from build123d import *

# Parameters (mm, degrees)
ESQUISSE2_W             = 100
ESQUISSE2_H             = 100
BOSS_EXTRU_1_DEPTH      = 100
ESQUISSE3_R             = 10
ENL_V_MAT_EXTRU_1_DEPTH = 101
ESQUISSE4_R             = 10
ENL_V_MAT_EXTRU_2_DEPTH = 101


with BuildPart() as part:
    # Esquisse2 → Boss.-Extru.1 (new body)
    with BuildSketch(Plane.XY):
        with Locations((-50, 50)):
            Rectangle(ESQUISSE2_W, ESQUISSE2_H)
    extrude(amount=BOSS_EXTRU_1_DEPTH)

    # Esquisse3 → Enlèv. mat.-Extru.1 (cut, through all)
    with BuildSketch(Plane.XY.offset(100)):
        with Locations((-50, 50)):
            Circle(ESQUISSE3_R)
    extrude(amount=-ENL_V_MAT_EXTRU_1_DEPTH, mode=Mode.SUBTRACT)

    # Esquisse4 → Enlèv. mat.-Extru.2 (cut, through all)
    with BuildSketch(Plane(origin=(0, 100, 0), x_dir=(1, 0, 0), z_dir=(0, 1, 0))):
        with Locations((-75, -25)):
            Circle(ESQUISSE4_R)
    extrude(amount=-ENL_V_MAT_EXTRU_2_DEPTH, mode=Mode.SUBTRACT)


solid = part.part
Model file for the job. Use its own axes, mm. Give positions to 0.01 mm unless a question says otherwise; leave off trailing zeros. Order: outer loops, then holes, each group sorted by start corner. A loop starts at its lowest first (then second) coordinate and runs counter-clockwise, first axis right, second up. Notation, with made-up numbers: M 69.5,18.25 L 80.5,18.25 A33 ccw 80.5,48.25 Z; hole C 12,50.5 d3. An arc over 180 degrees is marked long. Write item = value, one per line.
Q1. Cut at C-C, the plane y = 80. List the corners of the cut face in (x, z), then the cut area to 3 significant figures.
Derived:
outline = M -100,0 L 0,0 L 0,100 L -100,100 Z; hole C -75,25 d20
area = 9,690 mm2
Q2. Flat gauge pin, fed straight in: pin 1 (3 mm diameter, centred on x = -81.5, y = 86.5, fed in from -Z). Where does the tip first touch, or does it go through?
Derived:
pin_1 = 0
Q3. Cut at B-B, the plane x = -50. List the corners of the cut face in (y, z).
Derived:
outline = M 0,0 L 40,0 L 40,100 L 0,100 Z; M 60,0 L 100,0 L 100,100 L 60,100 Z
Q4. Cut at D-D, the plane z = 50. List the corners of the cut face in (x, y).
Derived:
outline = M -100,0 L 0,0 L 0,100 L -100,100 Z; hole C -50,50 d20
Q5. Drill centre lines: line 1 (X direction, y = 31, z = 25); line 2 (Z direction, x = -75, y = 34); line 3 (Y direction, x = -50, z = 38.5). Where is each one in solid material? Low to high. Write a range as [from, to].
Derived:
line_1 = [-100, -85], [-65, 0]
line_2 = [0, 15], [35, 100]
line_3 = [0, 40], [60, 100]
Q6. Two-plate mould, pull along X, no slides. Class faces 1 (the cylindrical face through (-85, 51, 25)), 2 (the flat face through (-51, 0, 49)), 3 (the cylindrical face through (-52.17, 40.24, 50.7)), 4 (the flat face through (0, 49, 49)): pulls with the +X half, pulls with the -X half, needs draft (parallel to the pull), parting line crosses it, or undercut.
Derived:
face_1 = undercut
face_2 = needs draft
face_3 = undercut
face_4 = pulls with the +X half
Q7. Cut at A-A, the plane z = 25. List the corners of the cut face in (x, y).
Derived:
outline = M -100,0 L -85,0 L -85,100 L -100,100 Z; M -65,0 L 0,0 L 0,100 L -65,100 Z; hole C -50,50 d20
